```python
from build123d import *

# Parameters (mm, degrees)
SKETCH_1_W          = 20
SKETCH_1_H          = 38
EXTRUDE_1_DEPTH     = 3
SKETCH_2_W          = 20
SKETCH_2_H          = 3
EXTRUDE_2_DEPTH     = 35
SKETCH_4_R          = 1.5
CUT_EXTRUDE_2_DEPTH = 10
SKETCH_6_R          = 8
CUT_EXTRUDE_4_DEPTH = 10
SKETCH_7_W          = 48.70277248
SKETCH_7_H          = 15.025597173
CUT_EXTRUDE_5_DEPTH = 17
SKETCH_8_W          = 23.770758151
SKETCH_8_H          = 7.865139004
CUT_EXTRUDE_6_DEPTH = 8
SKETCH_9_W          = 25.851926442
SKETCH_9_H          = 19.370122162
CUT_EXTRUDE_7_DEPTH = 1
SKETCH_10_W         = 62.66737892
SKETCH_10_H         = 43.463838198
CUT_EXTRUDE_8_DEPTH = 1


with BuildPart() as part:
    # 草图1 → 凸台-拉伸1 (new body)
    with BuildSketch(Plane.XY):
        Rectangle(SKETCH_1_W, SKETCH_1_H)
    extrude(amount=EXTRUDE_1_DEPTH)

    # 草图2 → 凸台-拉伸2 (add)
    with BuildSketch(Plane.XY.offset(3)):
        with Locations((0, -17.5)):
            Rectangle(SKETCH_2_W, SKETCH_2_H)
    extrude(amount=EXTRUDE_2_DEPTH)

    # 草图4 → 切除-拉伸2 (cut)
    with BuildSketch(Plane(origin=(0, -16, 0), x_dir=(1, 0, 0), z_dir=(0, 1, 0))):
        with Locations((-5, -13)):
            Circle(SKETCH_4_R)
        with Locations((5, -13)):
            Circle(SKETCH_4_R)
    extrude(amount=-CUT_EXTRUDE_2_DEPTH, mode=Mode.SUBTRACT)

    # 草图6 → 切除-拉伸4 (cut)
    with BuildSketch(Plane(origin=(0, 0, 0), x_dir=(-1, 0, 0), z_dir=(0, 0, -1))):
        with Locations((0, 1)):
            Circle(SKETCH_6_R)
    extrude(amount=-CUT_EXTRUDE_4_DEPTH, mode=Mode.SUBTRACT)

    # 草图7 → 切除-拉伸5 (cut)
    with BuildSketch(Plane.XY.offset(38)):
        with Locations((-7.483280409, -20.314408955)):
            Rectangle(SKETCH_7_W, SKETCH_7_H)
    extrude(amount=-CUT_EXTRUDE_5_DEPTH, mode=Mode.SUBTRACT)

    # 草图8 → 切除-拉伸6 (cut)
    with BuildSketch(Plane(origin=(0, 19, 0), x_dir=(1, 0, 0), z_dir=(0, 1, 0))):
        with Locations((-0.181621183, -1.317277333)):
            Rectangle(SKETCH_8_W, SKETCH_8_H)
    extrude(amount=-CUT_EXTRUDE_6_DEPTH, mode=Mode.SUBTRACT)

    # 草图9 → 切除-拉伸7 (cut)
    with BuildSketch(Plane(origin=(0, -16, 0), x_dir=(1, 0, 0), z_dir=(0, 1, 0))):
        with Locations((2.925963221, -12.685061081)):
            Rectangle(SKETCH_9_W, SKETCH_9_H)
    extrude(amount=-CUT_EXTRUDE_7_DEPTH, mode=Mode.SUBTRACT)

    # 草图10 → 切除-拉伸8 (cut)
    with BuildSketch(Plane(origin=(0, 0, 0), x_dir=(-1, 0, 0), z_dir=(0, 0, -1))):
        with Locations((0.038577245, -3.3946505)):
            Rectangle(SKETCH_10_W, SKETCH_10_H)
    extrude(amount=-CUT_EXTRUDE_8_DEPTH, mode=Mode.SUBTRACT)


solid = part.part
```
The model under review builds one solid part; all positions refer to its coordinate system, in mm. A direction names the side the tool comes from. Coordinates: 2 decimals unless noted, no trailing zeros. Write each loop counter-clockwise with the first axis right and the second up, starting at its lowest first coordinate (ties: lowest second). Pieces come first, ordered by that corner, then holes. Notation, with made-up numbers: (54, 9.25) - (102, 9.25) arc R23 ccw to (102, 29.25) - close; hole circle Ø2 at (-15, -8). An arc over 180 degrees is marked (long way). Answer in a Markdown table with one row per item. Add a question column.
Q1. Clearance check with flat-ended pins moving along their axes: pin 1 (3 mm diameter, centred on x = -5.5, y = 8, fed in from +Z); pin 2 (1 mm diameter, centred on x = -2.5, y = 6, fed in from -Z); pin 3 (10 mm diameter, centred on x = -4.5, z = 13.5, fed in from +Y). State where each tip first meets the part, or that it passes through.
Q2. Consider section C-C on x = 0. Give the boundary of the cut face in (y, z).
Q3. To check wall thickness, follow line 1 along X through (y, z) = (-18.05, 13); line 2 along Z through (x, y) = (-5, -17.5); line 3 along Y through (x, z) = (0, 1.8). State the ranges of each line that lie inside material, in increasing order. Write a range as from..to.
Q4. Consider section A-A on y = 1. Give the boundary of the cut face in (x, z).
Q5. Consider section B-B on z = 13. Give the boundary of the cut face in (x, y), then the cut area to 3 significant figures.
Q6. For faces 1 (the face through (0, -17, 12)), 2 (the face through (-2, -7, 1)), list the 3-axis set-ups (+Z, -Z, +X, -X, +Y, -Y) from which the entire face can be reached by the end or side of a thin tool; tool diameter is ignored.
Q7. Draft analysis for pull direction Z (two halves, no side actions). For faces 3 (the face through (0, -9, 3)), 4 (the face through (6.386, -17.986, 13.575)), 5 (the face through (-10, -10.7, 2.8)), state which applies: +Z half, -Z half, draft (parallel to the pull), parting line (faces both ways), or undercut.
Q8. Consider section D-D on x = 5. Give the boundary of the cut face in (y, z) (3 decimals).
Answers below:
| question | item | result |
|---|---|---|
| 1 | pin 1 | z = 3 |
| 1 | pin 2 | through |
| 1 | pin 3 | y = -17 |
| 2 | outline | (-19, 1) - (-7, 1) - (-7, 3) - (-17, 3) - (-17, 21) - (-19, 21) - close; (9, 1) - (11, 1) - (11, 3) - (9, 3) - close |
| 3 | line 1 | -10..-6.5, -3.5..3.5, 6.5..10 |
| 3 | line 2 | 1..11.5, 14.5..21 |
| 3 | line 3 | -19..-7, 9..11 |
| 4 | outline | (-10, 1) - (-8, 1) - (-8, 3) - (-10, 3) - close; (8, 1) - (10, 1) - (10, 3) - (8, 3) - close |
| 5 | outline | (-10, -19) - (-6.5, -19) - (-6.5, -17) - (-10, -17) - close; (-3.5, -19) - (3.5, -19) - (3.5, -17) - (-3.5, -17) - close; (6.5, -19) - (10, -19) - (10, -17) - (6.5, -17) - close |
| 5 | area | 28.0 mm² |
| 6 | face 1 | +Z, +X, -X, +Y |
| 6 | face 2 | -Z, +X, -X, +Y, -Y |
| 7 | face 3 | +Z half |
| 7 | face 4 | undercut |
| 7 | face 5 | draft |
| 8 | outline | (-19, 1) - (-5.245, 1) - (-5.245, 3) - (-17, 3) - (-17, 11.5) - (-19, 11.5) - close; (-19, 14.5) - (-17, 14.5) - (-17, 21) - (-19, 21) - close; (7.245, 1) - (11, 1) - (11, 3) - (7.245, 3) - close |
